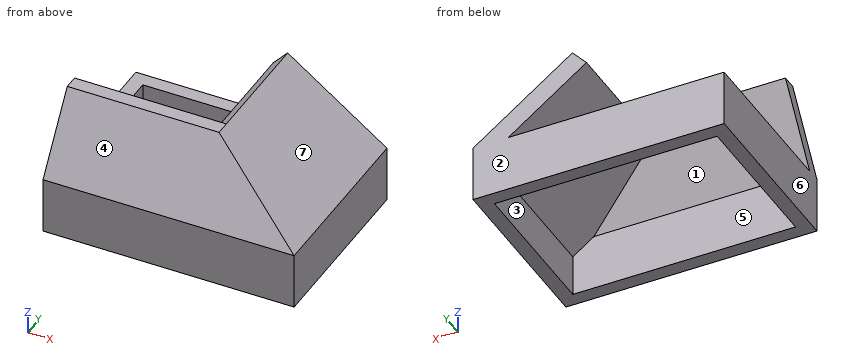
```python
from build123d import *

# Parameters (mm, degrees)
SKETCH1_W           = 17.7
SKETCH1_H           = 12.8
SKETCH1_W_2         = 15.7
SKETCH1_H_2         = 10.8
BOSS_EXTRUDE1_DEPTH = 4
BOSS_EXTRUDE2_DEPTH = 12.8
BOSS_EXTRUDE3_DEPTH = 17.7
CUT_EXTRUDE1_DEPTH  = 18.7
CUT_EXTRUDE3_REACH  = 19.7


with BuildPart() as part:
    # Sketch1 → Boss-Extrude1 (new body)
    with BuildSketch(Plane.XY):
        with Locations((-17.55, -7.7)):
            Rectangle(SKETCH1_W, SKETCH1_H)
        with Locations((-17.55, -7.7)):
            Rectangle(SKETCH1_W_2, SKETCH1_H_2, mode=Mode.SUBTRACT)
    extrude(amount=-BOSS_EXTRUDE1_DEPTH)

    # Sketch7 → Boss-Extrude2 (add)
    with BuildSketch(Plane.XZ.offset(14.1)):
        Polygon((-8.7, 0), (-15.7, 5.077748715), (-16.7, 4), (-9.7, -1.077748715), align=None)
    extrude(amount=-BOSS_EXTRUDE2_DEPTH)

    # Sketch11 → Boss-Extrude3 (add)
    with BuildSketch(Plane(origin=(-8.7, 0, -8.7), x_dir=(0, 0, 1), z_dir=(1, 0, 0))):
        Polygon((8.7, 13.1), (8.7, 14.1), (13.777748715, 10.756920169), (13.777748715, 9.756920169), align=None)
    extrude(amount=-BOSS_EXTRUDE3_DEPTH)

    # Sketch13 → Cut-Extrude1 (cut, through all)
    with BuildSketch(Plane(origin=(-8.7, 0, 0), x_dir=(0, 0, -1), z_dir=(1, 0, 0))):
        Polygon((-5.077748715, -10.756920169), (-5.077748715, -15.295870945), (0, -14.1), align=None)
    extrude(amount=-CUT_EXTRUDE1_DEPTH, mode=Mode.SUBTRACT)

    # Cut-Extrude3: up to this face of the body (flat: up to its plane)
    cut_extrude3_end = Plane(part.part.faces().sort_by_distance((-12.007460376, -6.410206852, 2.399207524))[0])
    # Sketch11<3> → Cut-Extrude3 (cut, up to the picked face)
    with BuildSketch(Plane(origin=(-8.7, 0, -8.7), x_dir=(0, 0, 1), z_dir=(1, 0, 0)), mode=Mode.PRIVATE) as cut_extrude3_sk1:
        Polygon((8.7, 13.1), (8.7, 14.1), (13.777748715, 10.756920169), (13.777748715, 9.756920169), align=None)
    cut_extrude3_tool1 = split(extrude(cut_extrude3_sk1.sketch, amount=-CUT_EXTRUDE3_REACH, mode=Mode.PRIVATE), bisect_by=cut_extrude3_end, keep=Keep.BOTH, mode=Mode.PRIVATE)
    add(cut_extrude3_tool1.solids().sort_by_distance((-8.7, -11.92846, 2.538874))[0], mode=Mode.SUBTRACT)


solid = part.part
```
Check sheet for the modelled part. Datum: model origin and axes. Units: mm. Face numbers are marked on the shaded views. A direction names the side the tool comes from. Round coordinates to 2 decimals unless told otherwise and drop trailing zeros. Order: outer loops, then holes, each group sorted by start corner. A loop starts at its lowest first (then second) coordinate and runs counter-clockwise, first axis right, second up. Notation, with made-up numbers: (64, 75) -> (113, 75) arc R34 cw to (113, 109) -> close; hole circle Ø10 at (-23.5, 12.25). An arc over 180 degrees is marked (long way). One line per item, written item: value. Start each with the question number.
Q1. Set-up check for the marked faces 1, 2 and 3: record each of +Z, -Z, +X, -X, +Y, -Y from which the full face is reachable in a straight line by a thin tool's end or side.
Q2. Gauge pin test, flat ends, axial feed: pin 1 Ø1.5 at (x, y) = (-20.5, -9.5) entering from -Z; pin 2 Ø1 at (y, z) = (-8.5, 3) entering from -X. Record the tip position at first contact, or that the pin passes through.
Q3. Cross-section at A-A (y = -9.25). Record the boundary of the cut face in (x, z), and give its area (3 significant figures).
Q4. Cross-section at D-D (y = -12). Record the boundary of the cut face in (x, z), and give its area (3 significant figures).
Q5. Cross-section at B-B (x = -21.75). Record the boundary of the cut face in (y, z), and give its area (3 significant figures).
Q6. Cross-section at C-C (z = -2.25). Record the boundary of the cut face in (x, y), and give its area (3 significant figures).
Q7. Mould release check, pull along X, two halves, no side actions. Record for the marked faces 4, 5, 6 and 7: pulls with the +X half, pulls with the -X half, needs draft (parallel to the pull), parting line crosses it, or undercut.
Q8. Thickness scan on line 1 (X direction, y = -7.25, z = -2.75); line 2 (Y direction, x = -20, z = -3.5); line 3 (X direction, y = -4.5, z = -0.5). Record the ranges inside material, lowest first.
Completed:
1. face 1: -X, +Y
1. face 2: +Z, -Z, +X, -X, +Y
1. face 3: -Z
2. pin 1: stops at z = 4.33
2. pin 2: stops at x = -16.01
3. outline: (-26.4, -4) -> (-25.4, -4) -> (-25.4, 0) -> (-26.4, 0) -> close; (-16.7, 4) -> (-9.7, -1.08) -> (-9.7, -4) -> (-8.7, -4) -> (-8.7, 0) -> (-15.7, 5.08) -> close
3. area: 20.1 mm²
4. outline: (-26.4, -4) -> (-25.4, -4) -> (-25.4, 0) -> (-26.4, 0) -> close; (-26.4, 1.67) -> (-13.49, 1.67) -> (-9.7, -1.08) -> (-9.7, -4) -> (-8.7, -4) -> (-8.7, 0) -> (-13.1, 3.19) -> (-26.4, 3.19) -> close
4. area: 34.7 mm²
5. outline: (-14.1, -4) -> (-13.1, -4) -> (-13.1, 0) -> (-9.76, 5.08) -> (-10.76, 5.08) -> (-14.1, 0) -> close; (-2.3, -4) -> (-1.3, -4) -> (-1.3, 0) -> (-2.3, 0) -> close
5. area: 13.1 mm²
6. outline: (-26.4, -14.1) -> (-8.7, -14.1) -> (-8.7, -1.3) -> (-26.4, -1.3) -> close; hole (-25.4, -13.1) -> (-9.7, -13.1) -> (-9.7, -2.3) -> (-25.4, -2.3) -> close
6. area: 57.0 mm²
7. face 4: needs draft
7. face 5: undercut
7. face 6: pulls with the -X half
7. face 7: pulls with the +X half
8. line 1: x = -26.4 to -25.4, -9.7 to -8.7
8. line 2: y = -14.1 to -13.1, -2.3 to -1.3
8. line 3: x = -26.4 to -25.4, -10.5 to -8.7
